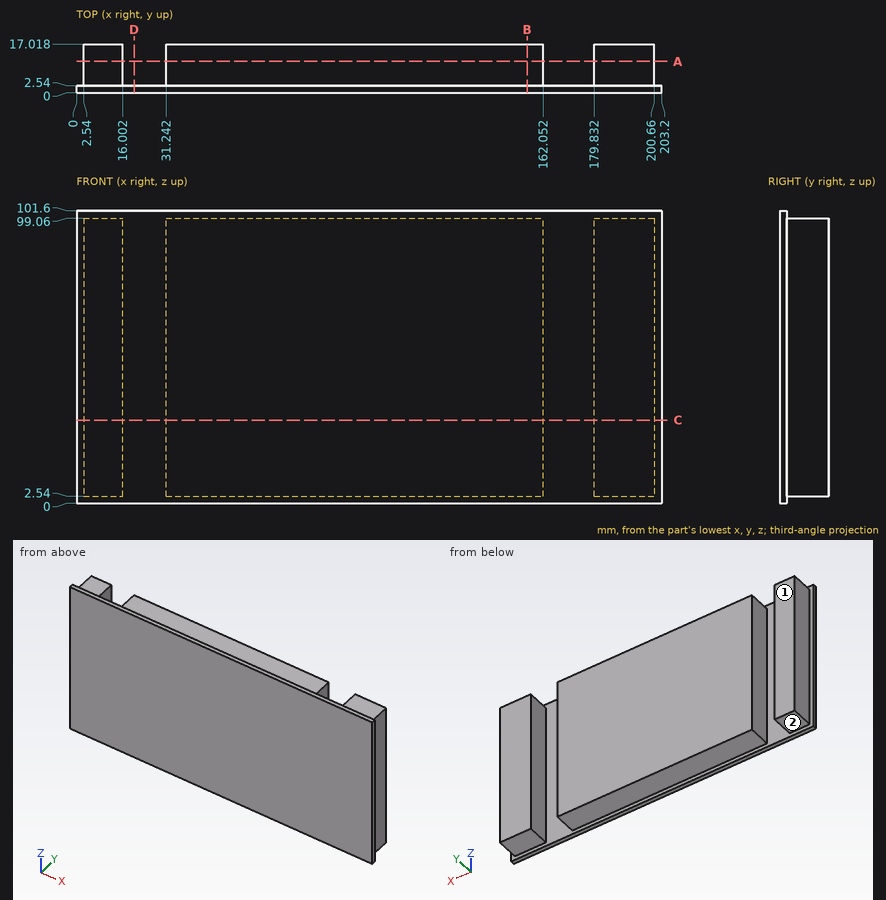
Geometry check sheet. Reference: drawing and pictorial views, mm from the part's lowest x, y, z. A direction names the side the tool comes from. Round coordinates to 2 decimals unless told otherwise and drop trailing zeros. Write each loop counter-clockwise with the first axis right and the second up, starting at its lowest first coordinate (ties: lowest second). Pieces come first, ordered by that corner, then holes. Notation, with made-up numbers: (-17.75, -36) -> (4.25, -36) arc R26 cw to (4.25, 2) -> close; hole circle Ø1 at (49.25, 3). An arc over 180 degrees is marked (long way). Answer as CSV lines item,"result". Start each with the question number.
1) Section check A-A on y = 11. Enter the section's corners in (x, z).
2) Tool access check on the marked faces 1 and 2. Record the directions out of +Z, -Z, +X, -X, +Y, -Y that give a thin tool (end or side, any length) a straight path to the whole face; none if there is none.
3) Section check C-C on z = 29. Enter the section's corners in (x, y), and give its area (3 significant figures).
4) Material ranges on line 1 (X direction, y = 14.75, z = 51); line 2 (Z direction, x = 134, y = 3.25); line 3 (Y direction, x = 27, z = 35), recorded low to high. Write a range as from..to.
5) Section check D-D on x = 20. Enter the section's corners in (y, z).
6) Section check B-B on x = 156.5. Enter the section's corners in (y, z), and give its area (3 significant figures).
7) Go/stop test with flat-tipped pins: P1, Ø7, axis at y = 8.5, z = 59, coming from the -X side; P2, Ø1.5, axis at x = 42, y = 14, coming from the +Z side; P3, Ø4.5, axis at x = 190.5, y = 10, coming from the -Z side. Record where each tip stops, or that it passes through.
Found:
1,outline,"(2.54, 2.54) -> (16, 2.54) -> (16, 99.06) -> (2.54, 99.06) -> close; (31.24, 2.54) -> (162.05, 2.54) -> (162.05, 99.06) -> (31.24, 99.06) -> close; (179.83, 2.54) -> (200.66, 2.54) -> (200.66, 99.06) -> (179.83, 99.06) -> close"
2,face 1,"+Z, -Z, +X, -X, +Y"
2,face 2,"-Z, +X, -X, +Y"
3,outline,"(0, 0) -> (203.2, 0) -> (203.2, 2.54) -> (200.66, 2.54) -> (200.66, 17.02) -> (179.83, 17.02) -> (179.83, 2.54) -> (162.05, 2.54) -> (162.05, 17.02) -> (31.24, 17.02) -> (31.24, 2.54) -> (16, 2.54) -> (16, 17.02) -> (2.54, 17.02) -> (2.54, 2.54) -> (0, 2.54) -> close"
3,area,"2,910 mm^2"
4,line 1,"x = 2.54..16, 31.24..162.05, 179.83..200.66"
4,line 2,"z = 2.54..99.06"
4,line 3,"y = 0..2.54"
5,outline,"(0, 0) -> (2.54, 0) -> (2.54, 101.6) -> (0, 101.6) -> close"
6,outline,"(0, 0) -> (2.54, 0) -> (2.54, 2.54) -> (17.02, 2.54) -> (17.02, 99.06) -> (2.54, 99.06) -> (2.54, 101.6) -> (0, 101.6) -> close"
6,area,"1,660 mm^2"
7,P1,"stops at x = 2.54"
7,P2,"stops at z = 99.06"
7,P3,"stops at z = 2.54"
